Source: CAD feature listing. Evaluate the final solid. Frame: model axes, mm. A direction names the side the tool comes from. Give positions to 0.01 mm unless a question says otherwise; leave off trailing zeros. Order: outer loops, then holes, each group sorted by start corner. A loop starts at its lowest first (then second) coordinate and runs counter-clockwise, first axis right, second up. Notation, with made-up numbers: (-38.75, 48) - (3.25, 48) arc R9 ccw to (3.25, 57) - close; hole circle Ø3 at (22, 84). An arc over 180 degrees is marked (long way). One line per item, written item: value. Start each with the question number.
from build123d import *

# Parameters (mm, degrees)
SKETCH1_W           = 25.4
SKETCH1_H           = 9.525
BOSS_EXTRUDE1_DEPTH = 12.7
SKETCH2_R           = 1.5875
SKETCH2_W           = 6.35
SKETCH2_H           = 6.35
CUT_EXTRUDE1_DEPTH  = 19.581211108
SKETCH4_R           = 1.308790008
CUT_EXTRUDE2_DEPTH  = 20.05


with BuildPart() as part:
    # Sketch1 → Boss-Extrude1 (new body)
    with BuildSketch(Plane.XY):
        Rectangle(SKETCH1_W, SKETCH1_H)
    extrude(amount=BOSS_EXTRUDE1_DEPTH)

    # Sketch2 → Cut-Extrude1 (cut, through all)
    with BuildSketch(Plane.XY.offset(12.7)):
        with Locations((0, -1.0287)):
            Circle(SKETCH2_R)
        with Locations((-9.525, 1.5875)):
            Rectangle(SKETCH2_W, SKETCH2_H)
        with Locations((9.525, 1.5875)):
            Rectangle(SKETCH2_W, SKETCH2_H)
    extrude(amount=-CUT_EXTRUDE1_DEPTH, mode=Mode.SUBTRACT)

    # Sketch4 → Cut-Extrude2 (cut, through all)
    with BuildSketch(Plane(origin=(0, -1.5875, 0), x_dir=(1, 0, 0), z_dir=(0, 1, 0))):
        with Locations(Location((9.525, -6.35, 0), (0, 0, 180))):
            Circle(SKETCH4_R)
        with Locations(Location((-9.525, -6.35, 0), (0, 0, 180))):
            Circle(SKETCH4_R)
    extrude(amount=-CUT_EXTRUDE2_DEPTH, mode=Mode.SUBTRACT)


solid = part.part
1. Set-up query: faces 1 (the flat face through (8, -1.588, 6)), 2 (the flat face through (-8, -1.588, 6)), 3 (the cylindrical face through (10.6, -3.2, 5.6)). Return all of +Z, -Z, +X, -X, +Y, -Y with unobstructed straight access to the full face (end or side cutting, diameter ignored); none if empty.
2. Section B-B on y = -2.25. Return the cut outline in (x, z) (3 decimals).
3. Contact query for flat-ended pins moving along their axis: pin 1 Ø2 at (x, z) = (-7, 11) entering from +Y; pin 2 Ø1.9 at (x, y) = (0, -1.03) entering from +Z; pin 3 Ø3 at (y, z) = (1.5, 5) entering from +X; pin 4 Ø3 at (x, z) = (-9, 4) entering from +Y. Output: stop coordinate, or through.
4. Ray query, L1, parallel to Y at x = 0, z = 9.25; L2, parallel to Y at x = -7, z = 7.75; L3, parallel to X at y = 4, z = 10.25. Return the intervals inside material, ascending.
5. Section A-A on x = 0. Return the cut outline in (y, z).
6. Section C-C on z = 6.35. Count the separate pieces of the cut face and the enclosed holes in it, then the cut area to 3 significant figures.
7. Draft query along X for faces 4 (the flat face through (0, 1, 12.7)), 5 (the cylindrical face through (0.73, -2.44, 6.44)), 6 (the flat face through (12.7, -3, 6)). Return one class per face: pulls with the +X half, pulls with the -X half, needs draft (parallel to the pull), parting line crosses it, or undercut.
Data:
1. face 1: +Z, -Z, +X, +Y
1. face 2: +Z, -Z, -X, +Y
1. face 3: +Y, -Y
2. outline: (-12.7, 0) - (-1.014, 0) - (-1.014, 12.7) - (-12.7, 12.7) - close; (1.014, 0) - (12.7, 0) - (12.7, 12.7) - (1.014, 12.7) - close; hole circle Ø2.618 at (-9.525, 6.35); hole circle Ø2.618 at (9.525, 6.35)
3. pin 1: stops at y = 4.76
3. pin 2: passes through
3. pin 3: stops at x = 6.35
3. pin 4: stops at y = -1.59
4. L1: y = -4.76 to -2.62, 0.56 to 4.76
4. L2: y = -4.76 to -1.59
4. L3: x = -6.35 to 6.35
5. outline: (-4.76, 0) - (-2.62, 0) - (-2.62, 12.7) - (-4.76, 12.7) - close; (0.56, 0) - (4.76, 0) - (4.76, 12.7) - (0.56, 12.7) - close
6. separate pieces: 3
6. enclosed holes: 1
6. area: 137 mm2
7. face 4: needs draft
7. face 5: undercut
7. face 6: pulls with the +X half
